```python
from build123d import *

# Parameters (mm, degrees)
SKETCH1_R           = 37.5
BOSS_EXTRUDE1_DEPTH = 3
SKETCH2_R           = 35
BOSS_EXTRUDE2_DEPTH = 11
SKETCH4_R           = 2.6
CUT_EXTRUDE2_DEPTH  = 55.849794895
SKETCH5_R           = 20
CUT_EXTRUDE3_DEPTH  = 55.849794895
SKETCH6_R           = 4.75
CUT_EXTRUDE4_DEPTH  = 3


with BuildPart() as part:
    # Sketch1 → Boss-Extrude1 (new body)
    with BuildSketch(Plane(origin=(0, 0, 0), x_dir=(1, 0, 0), z_dir=(0, 1, 0))):
        with Locations(Location((0, 0, 0), (0, 0, 270))):
            Circle(SKETCH1_R)
    extrude(amount=BOSS_EXTRUDE1_DEPTH)

    # Sketch2 → Boss-Extrude2 (add)
    with BuildSketch(Plane(origin=(0, 3, 0), x_dir=(1, 0, 0), z_dir=(0, 1, 0))):
        with Locations(Location((0, 0, 0), (0, 0, 270))):
            Circle(SKETCH2_R)
    extrude(amount=BOSS_EXTRUDE2_DEPTH)

    # Sketch4 → Cut-Extrude2 (cut, through all)
    with BuildSketch(Plane(origin=(0, 14, 0), x_dir=(1, 0, 0), z_dir=(0, 1, 0))):
        with Locations(Location((-16.069690242, 19.151111078, 0), (0, 0, 270))):
            Circle(SKETCH4_R)
        with Locations(Location((16.069690242, 19.151111078, 0), (0, 0, 270))):
            Circle(SKETCH4_R)
        with Locations(Location((16.069690242, -19.151111078, 0), (0, 0, 270))):
            Circle(SKETCH4_R)
        with Locations(Location((-16.069690242, -19.151111078, 0), (0, 0, 270))):
            Circle(SKETCH4_R)
    extrude(amount=-CUT_EXTRUDE2_DEPTH, mode=Mode.SUBTRACT)

    # Sketch5 → Cut-Extrude3 (cut, through all)
    with BuildSketch(Plane(origin=(0, 14, 0), x_dir=(1, 0, 0), z_dir=(0, 1, 0))):
        with Locations(Location((0, 0, 0), (0, 0, 270))):
            Circle(SKETCH5_R)
    extrude(amount=-CUT_EXTRUDE3_DEPTH, mode=Mode.SUBTRACT)

    # Sketch6 → Cut-Extrude4 (cut)
    with BuildSketch(Plane.XZ):
        with Locations(Location((16.069690242, -19.151111078, 0), (0, 0, 270))):
            Circle(SKETCH6_R)
        with Locations(Location((-16.069690242, -19.151111078, 0), (0, 0, 270))):
            Circle(SKETCH6_R)
        with Locations(Location((16.069690242, 19.151111078, 0), (0, 0, 270))):
            Circle(SKETCH6_R)
        with Locations(Location((-16.069690242, 19.151111078, 0), (0, 0, 270))):
            Circle(SKETCH6_R)
    extrude(amount=-CUT_EXTRUDE4_DEPTH, mode=Mode.SUBTRACT)


solid = part.part
```
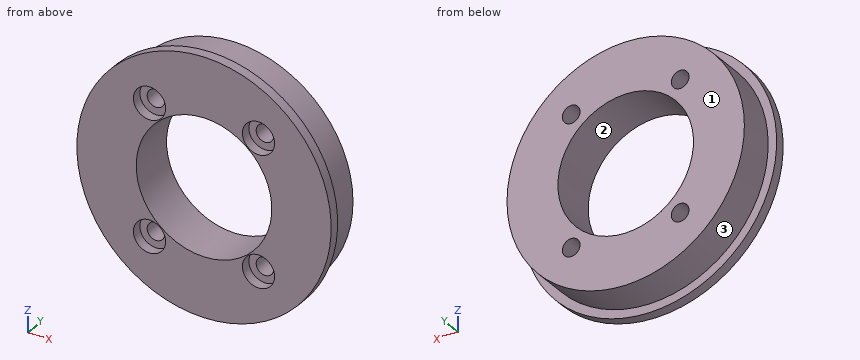
Geometry check sheet. Reference: the model listing, model coordinates, mm. Face numbers are marked on the shaded views. Round coordinates to 2 decimals unless told otherwise and drop trailing zeros. Loops run counter-clockwise (first coordinate to the right, second up) from the corner with the lowest first, then second, coordinate; pieces in that order, holes last. Notation, with made-up numbers: (-21, -16) - (38, -16) arc R24 cw to (38, 5) - close; hole circle Ø2 at (18.25, 29). An arc over 180 degrees is marked (long way). Use a Markdown table: item, result.
Q1. Cross-section at D-D on y = 1.25. Record the cut outline in (x, z).
Solutions:
| item | result |
|---|---|
| outline | circle Ø75 at (0, 0); hole circle Ø9.5 at (-16.07, -19.15); hole circle Ø9.5 at (-16.07, 19.15); hole circle Ø40 at (0, 0); hole circle Ø9.5 at (16.07, -19.15); hole circle Ø9.5 at (16.07, 19.15) |
Q2. Cross-section at C-C on x = -15. Record the cut outline in (y, z).
Solutions:
| item | result |
|---|---|
| outline | (0, -34.37) - (3, -34.37) - (3, -31.62) - (14, -31.62) - (14, -21.52) - (3, -21.52) - (3, -23.78) - (0, -23.78) - close; (0, -14.52) - (3, -14.52) - (3, -16.78) - (14, -16.78) - (14, -13.23) - (0, -13.23) - close; (0, 13.23) - (14, 13.23) - (14, 16.78) - (3, 16.78) - (3, 14.52) - (0, 14.52) - close; (0, 23.78) - (3, 23.78) - (3, 21.52) - (14, 21.52) - (14, 31.62) - (3, 31.62) - (3, 34.37) - (0, 34.37) - close |
Q3. Material ranges on line 1 (X direction, y = 4.75, z = 21.5); line 2 (X direction, y = 11.5, z = 17); line 3 (X direction, y = 3.25, z = 0), recorded low to high.
Solutions:
| item | result |
|---|---|
| line 1 | x = -27.62 to -17.18, -14.95 to 14.95, 17.18 to 27.62 |
| line 2 | x = -30.59 to -17.53, -14.61 to -10.54, 10.54 to 14.61, 17.53 to 30.59 |
| line 3 | x = -35 to -20, 20 to 35 |
Q4. Draft check along X on the marked faces 1, 2 and 3. Enter one of: released by +X, released by -X, zero draft, split by the parting line, or undercut.
Solutions:
| item | result |
|---|---|
| face 1 | zero draft |
| face 2 | undercut |
| face 3 | split by the parting line |
Q5. Cross-section at B-B on x = 0. Record the cut outline in (y, z), plus the area to 3 significant figures.
Solutions:
| item | result |
|---|---|
| outline | (0, -37.5) - (3, -37.5) - (3, -35) - (14, -35) - (14, -20) - (0, -20) - close; (0, 20) - (14, 20) - (14, 35) - (3, 35) - (3, 37.5) - (0, 37.5) - close |
| area | 435 mm2 |
Q6. Go/stop test with flat-tipped pins: P1, Ø8, axis at y = 9.5, z = -14, coming from the -X side; P2, Ø3, axis at x = 18, y = 10, coming from the -Z side; P3, Ø7, axis at x = -16.07, z = -19.15, coming from the -Y side. Record where each tip stops, or that it passes through.
Solutions:
| item | result |
|---|---|
| P1 | stops at x = -33.54 |
| P2 | stops at z = -30.87 |
| P3 | stops at y = 3 |
Q7. Cross-section at A-A on z = 0. Record the cut outline in (x, y), plus the area to 3 significant figures.
Solutions:
| item | result |
|---|---|
| outline | (-37.5, 0) - (-20, 0) - (-20, 14) - (-35, 14) - (-35, 3) - (-37.5, 3) - close; (20, 0) - (37.5, 0) - (37.5, 3) - (35, 3) - (35, 14) - (20, 14) - close |
| area | 435 mm2 |
